Could you check a few things on this drawing? It's one solid part, dimensions in mm from its lowest x, y, z. A direction names the side the tool comes from. Round coordinates to 2 decimals unless told otherwise and drop trailing zeros. Write each loop counter-clockwise with the first axis right and the second up, starting at its lowest first coordinate (ties: lowest second). Pieces come first, ordered by that corner, then holes. Notation, with made-up numbers: M -37,67 L -4,67 A22 cw -4,89 Z; hole C -26,70.25 d8. An arc over 180 degrees is marked long. One line per item, written item: value. Start each with the question number.
(1) I want a section at D-D on z = 41.5. Count the separate pieces of the cut face and the enclosed holes in it, and give its area (3 significant figures).
(2) If I drill on L1, parallel to X at y = 81, z = 38.5; L2, parallel to X at y = 5, z = 45.5; L3, parallel to Z at x = 87, y = 98.5, over which ranges is the centre line in solid material (lowest first)?
(3) I'm going to push flat-ended pins straight in: pin 1 Ø6.5 at (y, z) = (100.5, 48) entering from -X; pin 2 Ø4 at (x, y) = (88, 100) entering from +Z. Where does each tip first touch, or does it pass through?
(4) I want a section at C-C on y = 24.5. Please give me the cut outline in (x, z).
(5) Which directions (+Z, -Z, +X, -X, +Y, -Y) give clear straight access to the entire face, cutting with the end or side of a thin tool? Please do the marked faces 1 and 2.
(6) Thinking about a two-plate mould opening in X: for the marked faces 3, 4 and 5, which applies, released by +X, released by -X, zero draft, split by the parting line, or undercut?
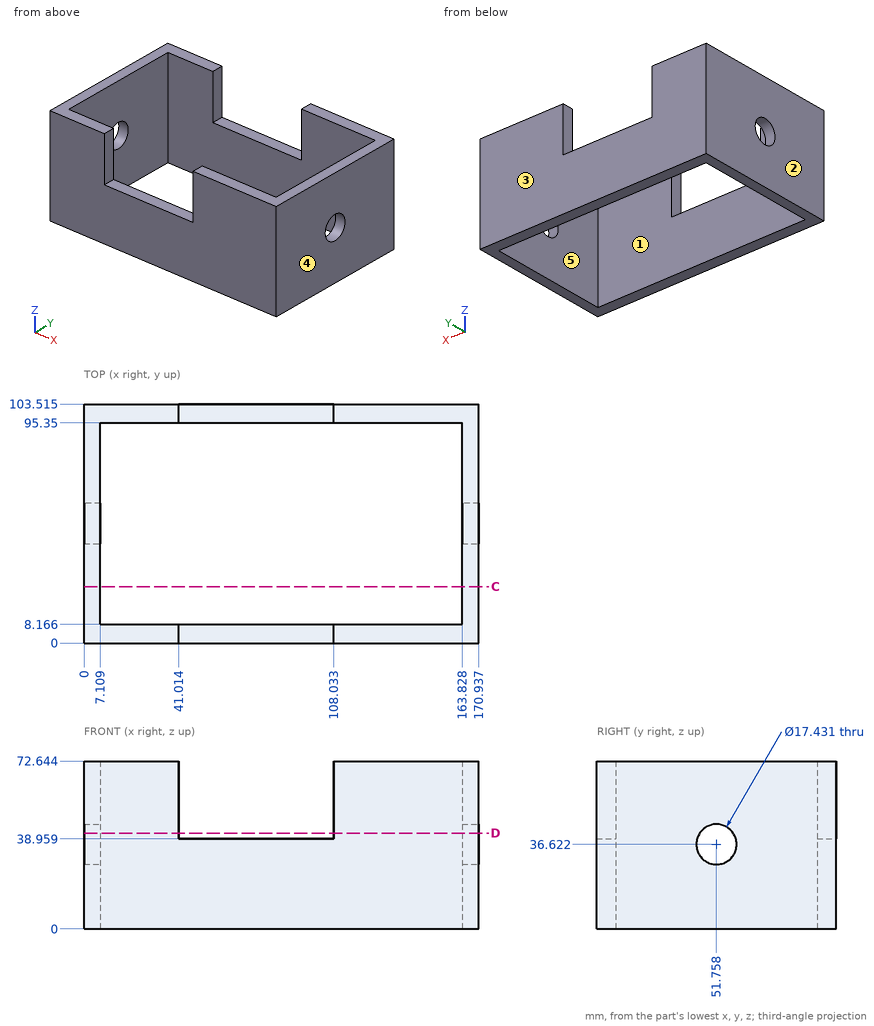
Found:
1. separate pieces: 4
1. enclosed holes: 0
1. area: 2,730 mm²
2. L1: x = 0 to 7.11, 163.83 to 170.94
2. L2: x = 0 to 41.01, 108.03 to 170.94
2. L3: z = 0 to 38.96
3. pin 1: stops at x = 0
3. pin 2: stops at z = 38.96
4. outline: M 0,0 L 7.11,0 L 7.11,72.64 L 0,72.64 Z; M 163.83,0 L 170.94,0 L 170.94,72.64 L 163.83,72.64 Z
5. face 1: +Z, -Z
5. face 2: +Z, -Z, -X, +Y, -Y
6. face 3: zero draft
6. face 4: released by +X
6. face 5: undercut
